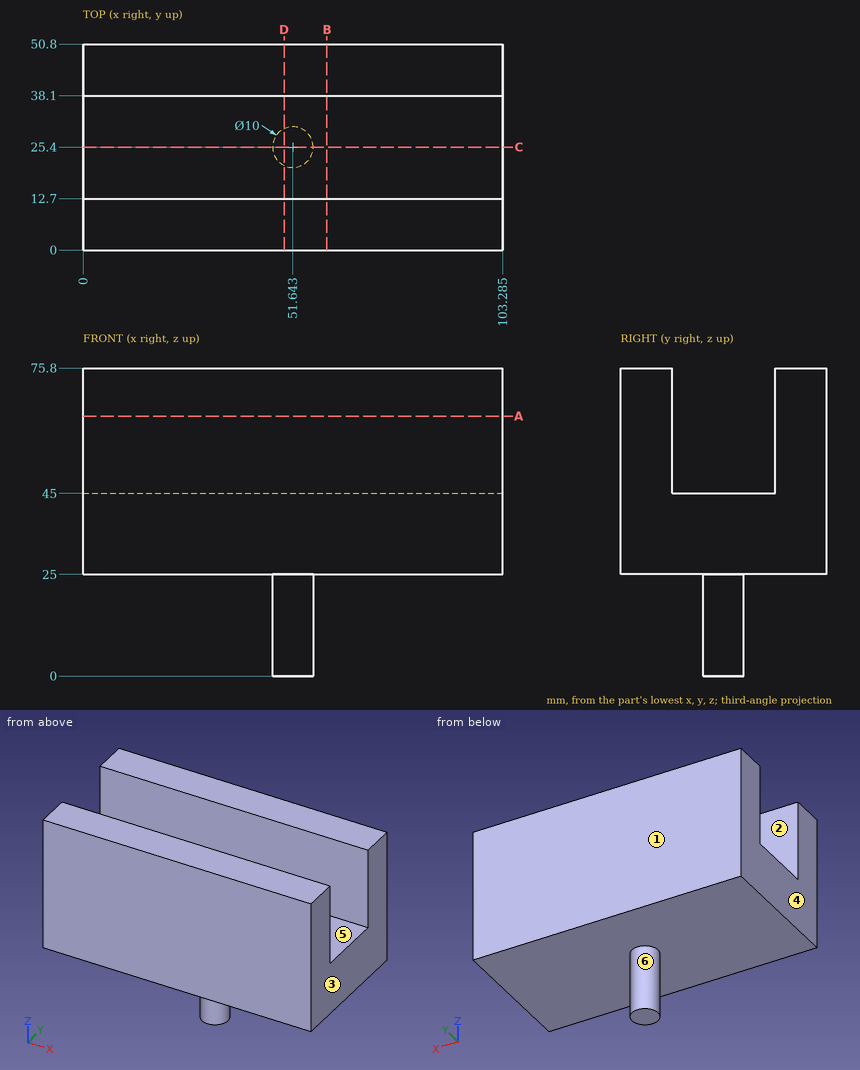
Verification items for this drawing (mm, ordinates from the low corner). A direction names the side the tool comes from. Coordinates: 2 decimals unless noted, no trailing zeros. Write each loop counter-clockwise with the first axis right and the second up, starting at its lowest first coordinate (ties: lowest second). Pieces come first, ordered by that corner, then holes. Notation, with made-up numbers: (-4, 83.25) - (25, 83.25) arc R11 cw to (25, 103.25) - close; hole circle Ø9 at (-30.75, -20.75). An arc over 180 degrees is marked (long way). One line per question, with ' | ' between items.
Item 1: Sectioned sample at B-B on x = 60. Record the boundary of the cut face in (y, z).
Determined:
outline: (0, 25) - (50.8, 25) - (50.8, 75.8) - (38.1, 75.8) - (38.1, 45) - (12.7, 45) - (12.7, 75.8) - (0, 75.8) - close
Item 2: Sectioned sample at D-D on x = 49.5. Record the boundary of the cut face in (y, z), plus the area to 3 significant figures.
Determined:
outline: (0, 25) - (20.88, 25) - (20.88, 0) - (29.92, 0) - (29.92, 25) - (50.8, 25) - (50.8, 75.8) - (38.1, 75.8) - (38.1, 45) - (12.7, 45) - (12.7, 75.8) - (0, 75.8) - close | area: 2,020 mm2
Item 3: Sectioned sample at A-A on z = 64. Record the boundary of the cut face in (x, y) (1 decimal).
Determined:
outline: (0, 0) - (103.3, 0) - (103.3, 12.7) - (0, 12.7) - close; (0, 38.1) - (103.3, 38.1) - (103.3, 50.8) - (0, 50.8) - close
Item 4: Mould release check, pull along Y, two halves, no side actions. Record for the marked faces 1, 2 and 3: pulls with the +Y half, pulls with the -Y half, needs draft (parallel to the pull), parting line crosses it, or undercut.
Determined:
face 1: pulls with the +Y half | face 2: undercut | face 3: needs draft
Item 5: Gauge pin test, flat end, axial feed: P1, Ø6, axis at x = 53, y = 40.5, coming from the -Z side. Record the tip position at first contact, or that the pin passes through.
Determined:
P1: stops at z = 25
Item 6: Access from +Z, -Z, +X, -X, +Y, -Y to the whole of each face (thin tool, end or side, straight path). Record for the marked faces 4, 5 and 6.
Determined:
face 4: +Z, -Z, -X, +Y, -Y | face 5: +Z, +X, -X | face 6: -Z
Item 7: Sectioned sample at C-C on y = 25.4. Record the boundary of the cut face in (x, z) (1 decimal).
Determined:
outline: (0, 25) - (46.6, 25) - (46.6, 0) - (56.6, 0) - (56.6, 25) - (103.3, 25) - (103.3, 45) - (0, 45) - close
Item 8: Thickness scan on line 1 (Y direction, x = 97, z = 57.5); line 2 (Z direction, x = 92.5, y = 36.5); line 3 (Z direction, x = 64, y = 8.5). Record the ranges inside material, lowest first. Write a range as [from, to].
Determined:
line 1: y = [0, 12.7], [38.1, 50.8] | line 2: z = [25, 45] | line 3: z = [25, 75.8]
